Build history of the part. All positions in model axes, mm. Give positions to 0.01 mm unless a question says otherwise; leave off trailing zeros. Loops run counter-clockwise (first coordinate to the right, second up) from the corner with the lowest first, then second, coordinate; pieces in that order, holes last. Notation, with made-up numbers: M 31,6.5 L 90,6.5 A25 cw 90,32.5 Z; hole C -12.5,42.25 d9. An arc over 180 degrees is marked long. Answer in a Markdown table with one row per item. Add a question column.
```python
from build123d import *

# Parameters (mm, degrees)
F0_W      = 110
F0_H      = 110
F1_DEPTH  = 5
F3_DEPTH  = 100
F4_SIZE   = 7
F6_DEPTH  = 5
F8_DEPTH  = 100
F9_R      = 3
F10_R     = 3
F11_R     = 5
F12_R     = 40
F13_DEPTH = 2
F14_R     = 40
F15_DEPTH = 2
F17_DEPTH = 200


with BuildPart() as f1:
    # F0 (on Top) → F1 (new body)
    with BuildSketch(Plane.XY):
        Rectangle(F0_W, F0_H)
    extrude(amount=F1_DEPTH)

    # F2 (on face) → F3 (join)
    with BuildSketch(Plane.XY.offset(5)):
        Polygon((-55, -45), (-55, -55), (-45, -55), (-45, -50), (-50, -50), (-50, -45), align=None)
        Polygon((45, -50), (45, -55), (55, -55), (55, -45), (50, -45), (50, -50), align=None)
        Polygon((50, 45), (55, 45), (55, 55), (45, 55), (45, 50), (50, 50), align=None)
        Polygon((-55, 45), (-50, 45), (-50, 50), (-45, 50), (-45, 55), (-55, 55), align=None)
    extrude(amount=F3_DEPTH)

    # F4
    f4_edges = [f1.edges().sort_by_distance(p)[0] for p in [
        (55, -55, 52.5),
        (55, 55, 52.5),
        (-55, -55, 52.5),
        (-55, 55, 52.5),
    ]]
    chamfer(f4_edges, length=F4_SIZE)

    # F5 (on face) → F6 (join)
    with BuildSketch(Plane(origin=(0, 0, 0), x_dir=(1, 0, 0), z_dir=(0, 0, -1))):
        Polygon((-55, -48), (-55, 48), (-86.8553390593, 16.1446609407), (-86.8553390593, -86.8553390593), (16.1446609407, -86.8553390593), (48, -55), (-48, -55), align=None)
    extrude(amount=-F6_DEPTH)

    # F7 (on face) → F8 (join)
    with BuildSketch(Plane.XY.offset(5)):
        with BuildLine():
            Line((-86.8553390593, -16.1446609407), (-55, -48))
            Line((-55, -48), (-55, -45))
            add(Edge.make_bspline(
                [(-55, -45), (-61.680716385, -38.545717713), (-73.8128115293, -26.9133031572), (-84.5587400556, -12.5278182858), (-85.5100929907, -5.3594725865), (-85.6892368288, -2.2746161558)],
                knots=[0, 0, 0, 0, 0.4166944434, 0.7503780711, 1, 1, 1, 1], degree=3))
            Line((-85.6892368288, -2.2746161558), (-85.6892368288, 84.628576657))
            Line((-85.6892368288, 84.628576657), (-52.0303300859, 50.9696699141))
            Line((-52.0303300859, 50.9696699141), (-50.9696699141, 52.0303300859))
            Line((-50.9696699141, 52.0303300859), (-84.628576657, 85.6892368288))
            Line((-84.628576657, 85.6892368288), (2.2746161558, 85.6892368288))
            add(Edge.make_bspline(
                [(45, 55), (38.545717713, 61.680716385), (26.9133031572, 73.8128115293), (12.5278182858, 84.5587400556), (5.3594725865, 85.5100929907), (2.2746161558, 85.6892368288)],
                knots=[0, 0, 0, 0, 0.4166944434, 0.7503780711, 1, 1, 1, 1], degree=3))
            Line((45, 55), (48, 55))
            Line((48, 55), (16.1446609407, 86.8553390593))
            Line((16.1446609407, 86.8553390593), (-86.8553390593, 86.8553390593))
            Line((-86.8553390593, 86.8553390593), (-86.8553390593, -16.1446609407))
        make_face()
    extrude(amount=F8_DEPTH)

    # F9
    f9_edges = [f1.edges().sort_by_distance(p)[0] for p in [
        (-50.96967, 52.03033, 55),
        (-52.03033, 50.96967, 55),
    ]]
    fillet(f9_edges, radius=F9_R)

    # F10
    f10_edges = [f1.edges().sort_by_distance(p)[0] for p in [
        (45, 55, 55),
        (-55, -45, 55),
        (-85.689237, 84.628577, 55),
        (-84.628577, 85.689237, 55),
    ]]
    fillet(f10_edges, radius=F10_R)

    # F11
    f11_edges = [f1.edges().sort_by_distance(p)[0] for p in [
        (-86.855339, -16.144661, 52.5),
        (16.144661, 86.855339, 52.5),
    ]]
    fillet(f11_edges, radius=F11_R)

    # F12 (on face) → F13 (cut)
    with BuildSketch(Plane(origin=(0, 86.8553390593, 0), x_dir=(-1, 0, 0), z_dir=(0, 1, 0))):
        with Locations((36.3908729653, 52.5)):
            Circle(F12_R)
    extrude(amount=-F13_DEPTH, mode=Mode.SUBTRACT)

    # F14 (on face) → F15 (cut)
    with BuildSketch(Plane(origin=(-86.8553390593, 0, 0), x_dir=(0, -1, 0), z_dir=(-1, 0, 0))):
        with Locations((-36.3908729653, 52.5)):
            Circle(F14_R)
    extrude(amount=-F15_DEPTH, mode=Mode.SUBTRACT)

    # F16 (on face) → F17 (cut)
    with BuildSketch(Plane(origin=(51.5, -51.5, 0), x_dir=(0.7071067812, 0.7071067812, 0), z_dir=(0.7071067812, -0.7071067812, 0))):
        Polygon((0, 105), (-74.4917392731, 105), (-74.4917392731, 4), (75.3377377987, 4), (75.3377377987, 105), (4.9497474683, 105), align=None)
    extrude(amount=-F17_DEPTH, mode=Mode.SUBTRACT)


solid = f1.part
```
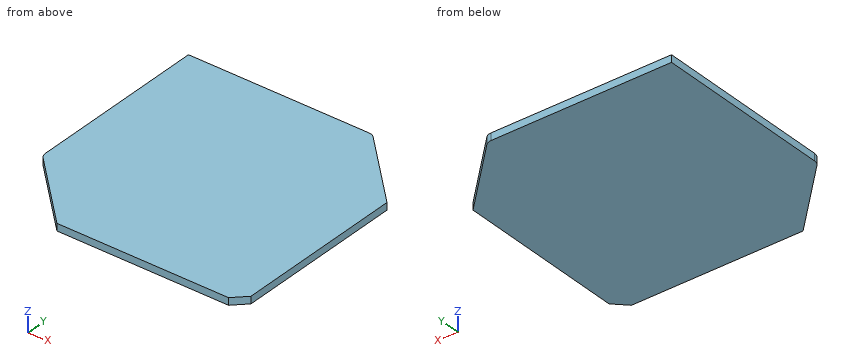
(1) Slice it at C-C, the plane x = 45.5. Give the cut face in (y, z), then the cut area to 3 significant figures.
(2) Slice it at A-A, the plane z = 1.45. Give the cut face in (x, y), then the cut area to 3 significant figures.
(3) Wall check: line 1 (X direction, y = -36.5, z = 3.1); line 2 (Y direction, x = 25, z = 3.4); line 3 (Y direction, x = -51, z = 0.6). Give the ranges that are in metal, low to high.
(4) Slice it at B-B, the plane y = -37.5. Give the cut face in (x, z).
Solution:
| question | item | result |
|---|---|---|
| 1 | outline | M -55,0 L 57.5,0 L 57.5,4 L -55,4 Z |
| 1 | area | 450 mm^2 |
| 2 | outline | M -86.86,-14.07 A5 ccw -85.39,-17.61 L -48,-55 L 48,-55 L 55,-48 L 55,48 L 17.61,85.39 A5 ccw 14.07,86.86 L -86.86,86.86 Z |
| 2 | area | 18,600 mm^2 |
| 3 | line 1 | -66.5 to 55 |
| 3 | line 2 | -55 to 78 |
| 3 | line 3 | -52 to 86.86 |
| 4 | outline | M -65.5,0 L 55,0 L 55,4 L -65.5,4 Z |
